from build123d import *

# Parameters (mm, degrees)
BOSS_EXTRUDE1_DEPTH = 10
SKETCH2_R           = 6
BOSS_EXTRUDE2_DEPTH = 10
SKETCH3_R           = 6
BOSS_EXTRUDE3_DEPTH = 10


with BuildPart() as part:
    # Sketch1 → Boss-Extrude1 (new body)
    with BuildSketch(Plane(origin=(0, 0, 0), x_dir=(1, 0, 0), z_dir=(0, 1, 0))):
        Polygon((57.735026919, 0), (28.867513459, 50), (-28.867513459, 50), (-57.735026919, 0), (-28.867513459, -50), (28.867513459, -50), align=None)
        Polygon((46.188021535, 0), (23.094010768, 40), (-23.094010768, 40), (-46.188021535, 0), (-23.094010768, -40), (23.094010768, -40), align=None, mode=Mode.SUBTRACT)
    extrude(amount=BOSS_EXTRUDE1_DEPTH)

    # Sketch2 → Boss-Extrude2 (add)
    with BuildSketch(Plane(origin=(-43.301270189, 0, 25), x_dir=(0.5000000000000071, 0, 0.8660254037844346), z_dir=(-0.8660254037844345, 0, 0.500000000000007))):
        with BuildLine():
            Line((15, 41.047826235), (15, 10))
            Line((15, 10), (-15, 10))
            Line((-15, 10), (-15, 41.047826235))
            ThreePointArc((-15, 41.047826235), (0, 56.047826235), (15, 41.047826235))
        make_face()
        with Locations((0, 41.047826235)):
            Circle(SKETCH2_R, mode=Mode.SUBTRACT)
    extrude(amount=-BOSS_EXTRUDE2_DEPTH)

    # Sketch3 → Boss-Extrude3 (add)
    with BuildSketch(Plane(origin=(43.301270189, 0, 25), x_dir=(0.4999999999999951, 0, -0.8660254037844415), z_dir=(0.8660254037844416, 0, 0.49999999999999517))):
        with BuildLine():
            Line((15, 41.047826235), (15, 10))
            Line((15, 10), (-15, 10))
            Line((-15, 10), (-15, 41.047826235))
            ThreePointArc((-15, 41.047826235), (0, 56.047826235), (15, 41.047826235))
        make_face()
        with Locations((0, 41.047826235)):
            Circle(SKETCH3_R, mode=Mode.SUBTRACT)
    extrude(amount=-BOSS_EXTRUDE3_DEPTH)


solid = part.part
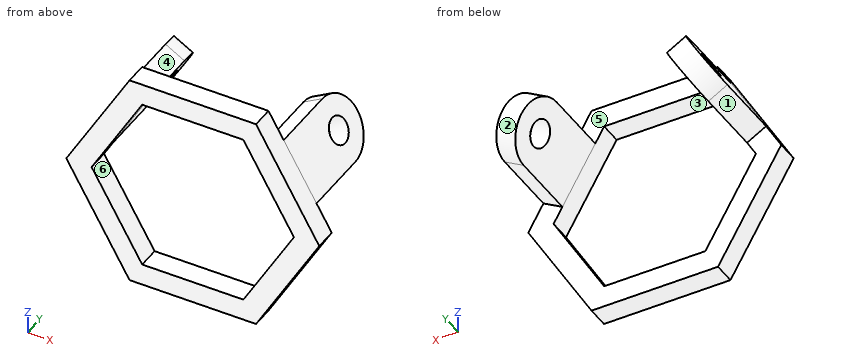
Build history of the part. All positions in model axes, mm. Face numbers are marked on the shaded views. A direction names the side the tool comes from. Round coordinates to 2 decimals unless told otherwise and drop trailing zeros. Loops run counter-clockwise (first coordinate to the right, second up) from the corner with the lowest first, then second, coordinate; pieces in that order, holes last. Notation, with made-up numbers: (-18.75, 25.5) -> (-10.75, 25.5) arc R23 cw to (-10.75, 37.5) -> close; hole circle Ø4 at (-39.5, 61.25). An arc over 180 degrees is marked (long way). Use CSV: the item, a comma, the result in double quotes. Start each with the question number.
Q1. Saw through at B-B on x = -13. Give the cut face in (y, z), and give its area (3 significant figures).
Q2. Flat gauge pins, fed straight in: pin 1 Ø18.5 at (x, z) = (-23, -23) entering from +Y; pin 2 Ø8 at (y, z) = (39.5, 14.5) entering from +X; pin 3 Ø4 at (x, y) = (-46, 21) entering from +Z; pin 4 Ø12 at (x, z) = (35, 10) entering from -Y. Where does each tip first touch, or does it go through?
Q3. Drill centre lines: L1, parallel to X at y = 20, z = 26.5; L2, parallel to Y at x = 34.5, z = -25.5; L3, parallel to X at y = 17, z = 17. Where is each one in solid material? Low to high.
Q4. Which spindle directions (+Z, -Z, +X, -X, +Y, -Y) get a long thin tool onto all of the face, cutting with end or side? Do the marked faces 1, 2 and 3. Say none if no direction does.
Q5. Saw through at A-A on y = 22. Give the cut face in (x, z).
Q6. Saw through at D-D on y = 44.5. Give the cut face in (x, z), and give its area (3 significant figures).
Q7. Saw through at C-C on y = 6.5. Give the cut face in (x, z), and give its area (3 significant figures).
Q8. Mould opens along Z. For the marked faces 4, 5 and 6 say: +Z half, -Z half, draft (parallel to the pull), parting line (faces both ways), or undercut.
Solutions:
1,outline,"(0, -50) -> (10, -50) -> (10, -40) -> (0, -40) -> close; (0, 40) -> (10, 40) -> (10, 50) -> (0, 50) -> close"
1,area,"200 mm^2"
2,pin 1,"stops at y = 10"
2,pin 2,"stops at x = 50.8"
2,pin 3,"stops at z = 23.79"
2,pin 4,"stops at y = 0"
3,L1,"x = -42.44 to -30.89, 30.89 to 42.44"
3,L2,"y = 0 to 10"
3,L3,"x = -47.92 to -36.37, 36.37 to 47.92"
4,face 1,"-Z, -X, +Y"
4,face 2,"+Y"
4,face 3,"+Y, -Y"
5,outline,"(-50.8, 12.01) -> (-42.14, 7.01) -> (-27.14, 32.99) -> (-35.8, 37.99) -> close; (27.14, 32.99) -> (42.14, 7.01) -> (50.8, 12.01) -> (35.8, 37.99) -> close"
6,outline,"(-50.6, 12.36) -> (-41.94, 7.36) -> (-37.09, 15.75) -> (-45.75, 20.75) -> close; (-40.85, 29.25) -> (-32.19, 24.25) -> (-27.34, 32.64) -> (-36, 37.64) -> close; (27.34, 32.64) -> (32.19, 24.25) -> (40.85, 29.25) -> (36, 37.64) -> close; (37.09, 15.75) -> (41.94, 7.36) -> (50.6, 12.36) -> (45.75, 20.75) -> close"
6,area,"388 mm^2"
7,outline,"(-57.74, 0) -> (-28.87, -50) -> (28.87, -50) -> (57.74, 0) -> (28.87, 50) -> (-28.87, 50) -> close; hole (-46.19, 0) -> (-23.09, -40) -> (23.09, -40) -> (46.19, 0) -> (23.09, 40) -> (-23.09, 40) -> close"
7,area,"3,120 mm^2"
8,face 4,"+Z half"
8,face 5,"draft"
8,face 6,"undercut"
